```python
from build123d import *

# Parameters (mm, degrees)
SKETCH2_R          = 1.5
CUT_EXTRUDE1_DEPTH = 41.620192023
CUT_EXTRUDE2_START = 10
SKETCH3_W          = 5
SKETCH3_H          = 5
CUT_EXTRUDE2_DEPTH = 31.620192023
SKETCH4_R          = 13.1
CUT_EXTRUDE3_DEPTH = 7.9


with BuildPart() as part:
    # Sketch1 → Revolve1 (revolve)
    with BuildSketch(Plane(origin=(0, 0, 0), x_dir=(0, 0, -1), z_dir=(1, 0, 0))):
        Polygon((0, 0), (25, 0), (5, 20), (0, 20), align=None)
    revolve(axis=Axis((0, 0, 0), (0, 1, 0)))

    # Sketch2 → Cut-Extrude1 (cut, through all)
    with BuildSketch(Plane(origin=(0, 0, 0), x_dir=(1, 0, 0), z_dir=(0, 1, 0))):
        with Locations(Location((0, 0, 0), (0, 0, 270))):
            Circle(SKETCH2_R)
    extrude(amount=CUT_EXTRUDE1_DEPTH, mode=Mode.SUBTRACT)

    # Sketch3 → Cut-Extrude2 (cut, through all)
    with BuildSketch(Plane(origin=(0, 0, 0), x_dir=(1, 0, 0), z_dir=(0, 1, 0)).offset(CUT_EXTRUDE2_START)):
        Rectangle(SKETCH3_W, SKETCH3_H)
    extrude(amount=CUT_EXTRUDE2_DEPTH, mode=Mode.SUBTRACT)

    # Sketch4 → Cut-Extrude3 (cut)
    with BuildSketch(Plane(origin=(0, 0, 0), x_dir=(1, 0, 0), z_dir=(0, 1, 0))):
        with Locations(Location((0, 0, 0), (0, 0, 270))):
            Circle(SKETCH4_R)
    extrude(amount=CUT_EXTRUDE3_DEPTH, mode=Mode.SUBTRACT)


solid = part.part
```
Part model, mm, in its own coordinate system. A direction names the side the tool comes from. Give positions to 0.01 mm unless a question says otherwise; leave off trailing zeros. Write each loop counter-clockwise with the first axis right and the second up, starting at its lowest first coordinate (ties: lowest second). Pieces come first, ordered by that corner, then holes. Notation, with made-up numbers: M 69.5,-19.5 L 111.5,-19.5 A30 ccw 111.5,5.5 Z; hole C -0.75,-24.5 d8. An arc over 180 degrees is marked long. Use CSV: the item, a comma, the result in double quotes.
Item 1: Pull direction X, two halves, no side cores. Call faces 4 (the face through (0, 15, -2.5)), 5 (the face through (8, 16.8, 1.8)), 6 (the face through (0, 20, -3)): +X half, -X half, draft (parallel to the pull), parting line (faces both ways), or undercut.
Taken from the geometry:
face 4,"undercut"
face 5,"parting line"
face 6,"draft"
Item 2: Pin check, flat tips, straight feed: P1, Ø4, axis at y = 17, z = -1, coming from the +X side; P2, Ø8, axis at x = -6.5, y = 7, coming from the +Z side; P3, Ø5, axis at x = 11, z = 5, coming from the +Y side. Stop position of each tip, or through.
Taken from the geometry:
P1,"stops at x = 9.96"
P2,"stops at z = 21.17"
P3,"stops at y = 15.42"
Item 3: Slice it at C-C on y = 13. Write the cut outline in (x, z).
Taken from the geometry:
outline,"C 0,0 d24; hole M -2.5,-2.5 L 2.5,-2.5 L 2.5,2.5 L -2.5,2.5 Z"
Item 4: Slice it at B-B on x = 0. Write the cut outline in (y, z).
Taken from the geometry:
outline,"M 0,-25 L 20,-5 L 20,-2.5 L 10,-2.5 L 10,-1.5 L 7.9,-1.5 L 7.9,-13.1 L 0,-13.1 Z; M 0,13.1 L 7.9,13.1 L 7.9,1.5 L 10,1.5 L 10,2.5 L 20,2.5 L 20,5 L 0,25 Z"
Item 5: Which spindle directions (+Z, -Z, +X, -X, +Y, -Y) get a long thin tool onto all of the face, cutting with end or side? Do faces 1 (the face through (11, 0, 11)), 2 (the face through (-3, 7.9, 0)), 3 (the face through (2.5, 15, 0)). Say none if no direction does.
Taken from the geometry:
face 1,"+Z, -Z, +X, -X, -Y"
face 2,"-Y"
face 3,"+Y"
Item 6: Slice it at D-D on y = 3.5. Write the cut outline in (x, z).
Taken from the geometry:
outline,"C 0,0 d43; hole C 0,0 d26.2"
Item 7: Slice it at A-A on z = 0. Write the cut outline in (x, y).
Taken from the geometry:
outline,"M -25,0 L -13.1,0 L -13.1,7.9 L -1.5,7.9 L -1.5,10 L -2.5,10 L -2.5,20 L -5,20 Z; M 1.5,7.9 L 13.1,7.9 L 13.1,0 L 25,0 L 5,20 L 2.5,20 L 2.5,10 L 1.5,10 Z"
Item 8: Drill centre lines: probe 1 along Z at (x, y) = (-7, 3); probe 2 along X at (y, z) = (3.25, -3.5); probe 3 along X at (y, z) = (4.5, 0). Where is each one in solid material? Low to high.
Taken from the geometry:
probe 1,"z = -20.86 to -11.07, 11.07 to 20.86"
probe 2,"x = -21.47 to -12.62, 12.62 to 21.47"
probe 3,"x = -20.5 to -13.1, 13.1 to 20.5"
